```python
from build123d import *

# Parameters (mm, degrees)
SKETCH1_W               = 150
SKETCH1_H               = 80
BOSS_EXTRUDE2_DEPTH     = 3
BOSS_EXTRUDE4_OUTLINE_W = 120
BOSS_EXTRUDE4_OUTLINE_H = 70
BOSS_EXTRUDE4_DEPTH     = 15
BOSS_EXTRUDE5_DEPTH     = 5
SKETCH6_W               = 110
SKETCH6_H               = 60
CUT_EXTRUDE1_DEPTH      = 5
SKETCH7_R               = 2.5
CUT_EXTRUDE2_DEPTH      = 5


# Read off the part's stored shape, not the designer's step: Boss-Extrude4
with BuildPart() as part:
    # Sketch1 → Boss-Extrude2 (new body)
    with BuildSketch(Plane.XY):
        with Locations((61.381224804, 30.24216319)):
            Rectangle(SKETCH1_W, SKETCH1_H)
    extrude(amount=BOSS_EXTRUDE2_DEPTH)

    # Boss-Extrude4 outline → Boss-Extrude4 (add)
    with BuildSketch(Plane(origin=(0, 0, 0), x_dir=(-1, 0, 0), z_dir=(0, 0, -1))):
        with Locations((-56.381224804, 25.24216319)):
            Rectangle(BOSS_EXTRUDE4_OUTLINE_W, BOSS_EXTRUDE4_OUTLINE_H)
    extrude(amount=BOSS_EXTRUDE4_DEPTH)

    # Sketch5 → Boss-Extrude5 (add)
    with BuildSketch(Plane(origin=(0, 0, 0), x_dir=(-1, 0, 0), z_dir=(0, 0, -1))):
        Polygon((-124.381224804, 19.24216319), (-124.381224804, 40.49216319), (-116.381224804, 40.49216319), (-116.381224804, -2.00783681), (-124.381224804, -2.00783681), align=None)
    extrude(amount=BOSS_EXTRUDE5_DEPTH)

    # Sketch6 → Cut-Extrude1 (cut)
    with BuildSketch(Plane(origin=(0, 0, -15), x_dir=(-1, 0, 0), z_dir=(0, 0, -1))):
        with Locations((-56.381224804, 25.24216319)):
            Rectangle(SKETCH6_W, SKETCH6_H)
    extrude(amount=-CUT_EXTRUDE1_DEPTH, mode=Mode.SUBTRACT)

    # Sketch7 → Cut-Extrude2 (cut)
    with BuildSketch(Plane(origin=(0, 0, 0), x_dir=(-1, 0, 0), z_dir=(0, 0, -1))):
        with Locations((-131.381224804, 65.24216319)):
            Circle(SKETCH7_R)
        with Locations((8.618775196, 65.24216319)):
            Circle(SKETCH7_R)
        with Locations((-131.381224804, -29.765126005)):
            Circle(SKETCH7_R)
        with Locations((8.618775196, -29.765126005)):
            Circle(SKETCH7_R)
    extrude(amount=-CUT_EXTRUDE2_DEPTH, mode=Mode.SUBTRACT)


solid = part.part
```
Geometry check sheet. Reference: the model listing, model coordinates, mm. A direction names the side the tool comes from. Give positions to 0.01 mm unless a question says otherwise; leave off trailing zeros. Order: outer loops, then holes, each group sorted by start corner. A loop starts at its lowest first (then second) coordinate and runs counter-clockwise, first axis right, second up. Notation, with made-up numbers: (51, 28) - (81, 28) arc R18 cw to (81, 32) - close; hole circle Ø1 at (60.5, 23.5). An arc over 180 degrees is marked (long way). Write item = value, one per line. Start each with the question number.
1) Section check C-C (z = -13.25). Enter the section's corners in (x, y), then the cut area to 3 significant figures.
2) Access from +Z, -Z, +X, -X, +Y, -Y to the whole of each face (thin tool, end or side, straight path). Record for faces 1 (the flat face through (-3.619, 25, -7)), 2 (the flat face through (120, -2.008, -2)), 3 (the flat face through (120, 40.492, -2)), 4 (the flat face through (57, 55.242, -13)).
3) Draft check along X on faces 5 (the cylindrical face through (130.228, 63.024, 1.479)), 6 (the flat face through (-13.619, 30, 1)), 7 (the flat face through (136.381, 30, 1)), 8 (the flat face through (120, 20, -5)). Enter one of: released by +X, released by -X, zero draft, split by the parting line, or undercut.
4) Section check A-A (y = 31.5). Enter the section's corners in (x, z).
5) Section check B-B (x = 76.5). Enter the section's corners in (y, z).
6) Section check D-D (y = 57). Enter the section's corners in (x, z).
7) Scan lines: L1, parallel to X at y = 47, z = -14; L2, parallel to Y at x = 11, z = -14; L3, parallel to Z at x = 107.5, y = 49. Record each from-to range of solid material in increasing order.
8) Gauge pin test, flat ends, axial feed: pin 1 Ø8 at (y, z) = (2.5, -5) entering from -X; pin 2 Ø2.5 at (x, z) = (69.5, -12) entering from +Y; pin 3 Ø9 at (x, y) = (121.5, 17.5) entering from -Z. Record the tip position at first contact, or that the pin passes through.
Geometry check:
q1.outline = (-3.62, -9.76) - (116.38, -9.76) - (116.38, 60.24) - (-3.62, 60.24) - close; hole (1.38, -4.76) - (111.38, -4.76) - (111.38, 55.24) - (1.38, 55.24) - close
q1.area = 1,800 mm2
q2.face_1 = -Z, -X, +Y, -Y
q2.face_2 = -Z, +X, -Y
q2.face_3 = -Z, +X, +Y
q2.face_4 = -Z
q3.face_5 = undercut
q3.face_6 = released by -X
q3.face_7 = released by +X
q3.face_8 = zero draft
q4.outline = (-13.62, 0) - (-3.62, 0) - (-3.62, -15) - (1.38, -15) - (1.38, -10) - (111.38, -10) - (111.38, -15) - (116.38, -15) - (116.38, -5) - (124.38, -5) - (124.38, 0) - (136.38, 0) - (136.38, 3) - (-13.62, 3) - close
q5.outline = (-9.76, -15) - (-4.76, -15) - (-4.76, -10) - (55.24, -10) - (55.24, -15) - (60.24, -15) - (60.24, 0) - (70.24, 0) - (70.24, 3) - (-9.76, 3) - close
q6.outline = (-13.62, 0) - (-3.62, 0) - (-3.62, -15) - (116.38, -15) - (116.38, 0) - (136.38, 0) - (136.38, 3) - (-13.62, 3) - close
q7.L1 = -3.62 to 1.38, 111.38 to 116.38
q7.L2 = -9.76 to -4.76, 55.24 to 60.24
q7.L3 = -10 to 3
q8.pin_1 = -3.62
q8.pin_2 = 60.24
q8.pin_3 = -5
